```python
from build123d import *

# Parameters (mm, degrees)
CROQUIS1_R              = 21
SALIENTE_EXTRUIR1_DEPTH = 49.5
CROQUIS3_R              = 3.9
CORTAR_EXTRUIR1_DEPTH   = 50.5
CROQUIS4_R              = 17.272
SALIENTE_EXTRUIR2_DEPTH = 7.5
CROQUIS5_R              = 3.9
CORTAR_EXTRUIR2_DEPTH   = 7.5
CROQUIS6_R              = 7.95
CORTAR_EXTRUIR3_DEPTH   = 6.35
CROQUIS7_R              = 7.95
CORTAR_EXTRUIR4_DEPTH   = 6.35


with BuildPart() as part:
    # Croquis1 → Saliente-Extruir1 (new body)
    with BuildSketch(Plane.XY):
        Circle(CROQUIS1_R)
    extrude(amount=SALIENTE_EXTRUIR1_DEPTH)

    # Croquis3 → Cortar-Extruir1 (cut, through all)
    with BuildSketch(Plane(origin=(0, 0, 0), x_dir=(-1, 0, 0), z_dir=(0, 0, -1))):
        Circle(CROQUIS3_R)
    extrude(amount=-CORTAR_EXTRUIR1_DEPTH, mode=Mode.SUBTRACT)

    # Croquis4 → Saliente-Extruir2 (add)
    with BuildSketch(Plane(origin=(0, 0, 0), x_dir=(-1, 0, 0), z_dir=(0, 0, -1))):
        Circle(CROQUIS4_R)
    extrude(amount=SALIENTE_EXTRUIR2_DEPTH)

    # Croquis5 → Cortar-Extruir2 (cut)
    with BuildSketch(Plane(origin=(0, 0, -7.5), x_dir=(-1, 0, 0), z_dir=(0, 0, -1))):
        Circle(CROQUIS5_R)
    extrude(amount=-CORTAR_EXTRUIR2_DEPTH, mode=Mode.SUBTRACT)

    # Croquis6 → Cortar-Extruir3 (cut)
    with BuildSketch(Plane(origin=(0, 0, -7.5), x_dir=(-1, 0, 0), z_dir=(0, 0, -1))):
        Circle(CROQUIS6_R)
    extrude(amount=-CORTAR_EXTRUIR3_DEPTH, mode=Mode.SUBTRACT)

    # Croquis7 → Cortar-Extruir4 (cut)
    with BuildSketch(Plane.XY.offset(49.5)):
        Circle(CROQUIS7_R)
    extrude(amount=-CORTAR_EXTRUIR4_DEPTH, mode=Mode.SUBTRACT)


solid = part.part
```
For this review, take the finished solid that the model builds, in its own axes (mm). A direction names the side the tool comes from. Round coordinates to 2 decimals unless told otherwise and drop trailing zeros. Write each loop counter-clockwise with the first axis right and the second up, starting at its lowest first coordinate (ties: lowest second). Pieces come first, ordered by that corner, then holes.
1) Insertion check: pin 1 Ø10 at (y, z) = (-6, 4.5) entering from +X; pin 2 Ø5 at (x, y) = (2.5, -3.5) entering from +Z; pin 3 Ø1 at (x, z) = (12.5, 42) entering from +Y; pin 4 Ø10 at (x, y) = (7, 16.5) entering from -Z. Each pin has a flat end and moves straight along its axis. Give the tip position at first contact, or say it passes through.
Answer below:
pin 1: stops at x = 20.98
pin 2: stops at z = 43.15
pin 3: stops at y = 17.23
pin 4: stops at z = -7.5
2) For line 1 along Y through (x, z) = (0, 46.25); line 2 along Y through (x, z) = (0, 16); line 3 along Z through (x, y) = (18, 10), list the stretches that pass through material, from the lowest coordinate up.
Answer below:
line 1: y = -21 to -7.95, 7.95 to 21
line 2: y = -21 to -3.9, 3.9 to 21
line 3: z = 0 to 49.5
3) Take a section at A-A on x = 0. Give the boundary of the cut face in (y, z), then the cut area to 3 significant figures.
Answer below:
outline: (-21, 0) - (-17.27, 0) - (-17.27, -7.5) - (-7.95, -7.5) - (-7.95, -1.15) - (-3.9, -1.15) - (-3.9, 43.15) - (-7.95, 43.15) - (-7.95, 49.5) - (-21, 49.5) - close; (3.9, -1.15) - (7.95, -1.15) - (7.95, -7.5) - (17.27, -7.5) - (17.27, 0) - (21, 0) - (21, 49.5) - (7.95, 49.5) - (7.95, 43.15) - (3.9, 43.15) - close
area: 1,790 mm2
4) Take a section at D-D on y = -9.5. Give the boundary of the cut face in (x, z).
Answer below:
outline: (-18.73, 0) - (-14.42, 0) - (-14.42, -7.5) - (14.42, -7.5) - (14.42, 0) - (18.73, 0) - (18.73, 49.5) - (-18.73, 49.5) - close
5) Mouldability with a two-part tool opening along X and no side actions: class faces 1 (the face through (2.248, 17.125, -3.698)), 2 (the face through (1.72, -7.76, -4.37)), 3 (the face through (-5, -17, 0)) as +X half, -X half, draft (parallel to the pull), parting line (faces both ways), or undercut.
Answer below:
face 1: parting line
face 2: undercut
face 3: draft
6) Take a section at C-C on z = -3. Give the boundary of the cut face in (x, y).
Answer below:
outline: circle Ø34.54 at (0, 0); hole circle Ø15.9 at (0, 0)
7) Machinability: for faces 4 (the face through (4, -2, -1.15)), 5 (the face through (-3.6, -7.4, -7.5)), 6 (the face through (-4, -2, 43.15)), which of the approach directions +Z, -Z, +X, -X, +Y, -Y give a long, thin tool a straight path to every point of the face, cutting with its end or side? Answer none if there is none.
Answer below:
face 4: -Z
face 5: -Z, +X, -X, +Y, -Y
face 6: +Z
